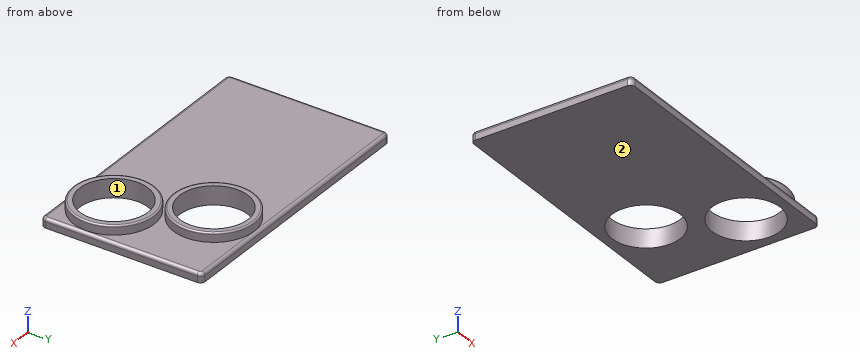
from build123d import *

# Parameters (mm, degrees)
F0_R         = 82.55
F0_R_2       = 69.85
F1_DEPTH     = 38.1
F0_W         = 558.8
F0_H         = 330.2
F2_DEPTH     = 19.05
F3_R         = 6.34999
F4_T1_DEPTH  = 42.8625
F4_T4_ANGLE  = 90
F4_T6_ANGLE  = 90
F4_T8_ANGLE  = 90
F4_T10_ANGLE = 90
F5_R         = 3.175


# Not quite as in the source:
# - a fillet or chamfer that OpenCascade refuses, or shapes differently, is made with other operations: its cross-section is extruded or revolved along the edge and cut away or added
# - a fillet or chamfer is up to 0.001 mm smaller than in the source, because OpenCascade refuses the exact size


with BuildPart() as f1:
    # F0 (on Top) → F1 (new body)
    with BuildSketch(Plane.XY):
        with Locations((393.7, 241.3)):
            Circle(F0_R)
        with Locations((393.7, 241.3)):
            Circle(F0_R_2, mode=Mode.SUBTRACT)
    extrude(amount=F1_DEPTH)



with BuildPart() as f1b:
    # F0 (on Top) → F1, piece 2 (new body)
    with BuildSketch(Plane.XY):
        with Locations((469.9, 88.9)):
            Circle(F0_R)
        with Locations((469.9, 88.9)):
            Circle(F0_R_2, mode=Mode.SUBTRACT)
    extrude(amount=F1_DEPTH)


with BuildPart() as f1_1:
    add(f1.part)

    add(f1b.part)  # F2 merges F1b
    # F0 (on Top) → F2 (join)
    with BuildSketch(Plane.XY):
        with Locations((279.4, 165.1)):
            Rectangle(F0_W, F0_H)
        with Locations((469.9, 88.9)):
            Circle(F0_R, mode=Mode.SUBTRACT)
        with Locations((393.7, 241.3)):
            Circle(F0_R, mode=Mode.SUBTRACT)
    extrude(amount=F2_DEPTH)

    # F3 (radius 6.35 in the source; OpenCascade refuses exactly that, so slightly less here)
    f3_edges = [f1_1.edges().sort_by_distance(p)[0] for p in [
        (0, 165.1, 19.05),
        (279.4, 330.2, 19.05),
        (279.4, 0, 19.05),
        (558.8, 165.1, 19.05),
    ]]
    fillet(f3_edges, radius=F3_R)

    # F4: fillet of radius 9.525 on 4 edges, made by hand

    # F4_s2 → F4_t1 (cut)
    with BuildSketch(Plane.XY.offset(-23.8125)):
        with BuildLine():
            ThreePointArc((0, 9.525), (2.7898079092, 2.7898079092), (9.525, 0))
            Line((9.525, 0), (0, 0))
            Line((0, 0), (0, 9.525))
        make_face()
        with BuildLine():
            ThreePointArc((549.275, 0), (556.0101920908, 2.7898079092), (558.8, 9.525))
            Line((558.8, 9.525), (558.8, 0))
            Line((558.8, 0), (549.275, 0))
        make_face()
        with BuildLine():
            ThreePointArc((549.275, 330.2), (556.0101920908, 327.4101920908), (558.8, 320.675))
            Line((558.8, 320.675), (558.8, 330.2))
            Line((558.8, 330.2), (549.275, 330.2))
        make_face()
        with BuildLine():
            ThreePointArc((0, 320.675), (2.7898079092, 327.4101920908), (9.525, 330.2))
            Line((9.525, 330.2), (0, 330.2))
            Line((0, 330.2), (0, 320.675))
        make_face()
    extrude(amount=F4_T1_DEPTH, mode=Mode.SUBTRACT)

    # F4_s3 → F4_t4 (revolve, cut)
    with BuildSketch(Plane.YZ.offset(9.525)):
        with BuildLine():
            ThreePointArc((323.85001, 19.05), (328.3401309895, 17.1901309895), (330.2, 12.70001))
            Line((330.2, 12.70001), (330.2, 19.05))
            Line((330.2, 19.05), (323.85001, 19.05))
        make_face()
    revolve(axis=Axis((9.525, 320.675, 19.05), (0, 0, 1)), revolution_arc=F4_T4_ANGLE, mode=Mode.SUBTRACT)

    # F4_s5 → F4_t6 (revolve, cut)
    with BuildSketch(Plane.XZ.offset(-320.675)):
        with BuildLine():
            ThreePointArc((552.45001, 19.05), (556.9401309895, 17.1901309895), (558.8, 12.70001))
            Line((558.8, 12.70001), (558.8, 19.05))
            Line((558.8, 19.05), (552.45001, 19.05))
        make_face()
    revolve(axis=Axis((549.275, 320.675, 19.05), (0, 0, 1)), revolution_arc=F4_T6_ANGLE, mode=Mode.SUBTRACT)

    # F4_s7 → F4_t8 (revolve, cut)
    with BuildSketch(Plane.YZ.offset(549.275)):
        with BuildLine():
            ThreePointArc((6.34999, 19.05), (1.8598690105, 17.1901309895), (0, 12.70001))
            Line((0, 12.70001), (0, 19.05))
            Line((0, 19.05), (6.34999, 19.05))
        make_face()
    revolve(axis=Axis((549.275, 9.525, 19.05), (0, 0, 1)), revolution_arc=F4_T8_ANGLE, mode=Mode.SUBTRACT)

    # F4_s9 → F4_t10 (revolve, cut)
    with BuildSketch(Plane.XZ.offset(-9.525)):
        with BuildLine():
            ThreePointArc((6.34999, 19.05), (1.8598690105, 17.1901309895), (0, 12.70001))
            Line((0, 12.70001), (0, 19.05))
            Line((0, 19.05), (6.34999, 19.05))
        make_face()
    revolve(axis=Axis((9.525, 9.525, 19.05), (0, 0, 1)), revolution_arc=F4_T10_ANGLE, mode=Mode.SUBTRACT)

    # F5
    f5_edges = [f1_1.edges().sort_by_distance(p)[0] for p in [
        (387.35, 88.9, 38.1),
        (311.15, 241.3, 38.1),
    ]]
    fillet(f5_edges, radius=F5_R)


solid = f1_1.part
Work out the finished part from the listing and answer in its coordinate system (mm). Face numbers are marked on the shaded views. Coordinates: 2 decimals unless noted, no trailing zeros. Write each loop counter-clockwise with the first axis right and the second up, starting at its lowest first coordinate (ties: lowest second). Pieces come first, ordered by that corner, then holes.
1. Consider line 1 along X through (y, z) = (238.5, 20); line 2 along Y through (x, z) = (393.7, 24); line 3 along Z through (x, y) = (337, 123.5). Determine where each line is inside the solid, lowest interval first.
Results list:
line 1: x = 311.2 to 323.91, 463.49 to 476.2
line 2: y = 57.15 to 120.65, 158.75 to 171.45, 311.15 to 323.85
line 3: z = 0 to 19.05
2. The part is cut by section C-C, the plane x = 38.5. Write down the section's boundary in (y, z), and give its area (3 significant figures).
Results list:
outline: (0, 0) - (330.2, 0) - (330.2, 12.7) arc R6.35 ccw to (323.85, 19.05) - (6.35, 19.05) arc R6.35 ccw to (0, 12.7) - close
area: 6,270 mm2
3. For a pull along X with two mould halves and no side action, classify the marked faces 1 and 2 as +X half, -X half, draft (parallel to the pull), parting line (faces both ways), or undercut.
Results list:
face 1: undercut
face 2: draft
4. Flat-ended cylindrical pins translate along their axes: pin 1 (1 mm diameter, centred on x = 176, z = 14, fed in from +Y); pin 2 (2 mm diameter, centred on y = 230.5, z = 28, fed in from -X); pin 3 (3 mm diameter, centred on x = 350.5, z = 17.5, fed in from -Y); pin 4 (5 mm diameter, centred on x = 190.5, z = 24, fed in from +Y). Find the tip coordinate at first contact, or state that the pin passes through.
Results list:
pin 1: stops at y = 330.15
pin 2: stops at x = 311.73
pin 3: stops at y = 0.92
pin 4: passes through
5. The part is cut by section A-A, the plane y = 241.3. Write down the section's boundary in (x, z) (3 decimals), and give its area (3 significant figures).
Results list:
outline: (0, 0) - (323.85, 0) - (323.85, 38.1) - (314.325, 38.1) arc R3.175 ccw to (311.15, 34.925) - (311.15, 19.05) - (6.35, 19.05) arc R6.35 ccw to (0, 12.7) - close; (463.55, 0) - (558.8, 0) - (558.8, 12.7) arc R6.35 ccw to (552.45, 19.05) - (476.25, 19.05) - (476.25, 34.925) arc R3.175 ccw to (473.075, 38.1) - (463.55, 38.1) - close
area: 8,450 mm2
6. The part is cut by section B-B, the plane z = 6. Write down the section's boundary in (x, y) (3 decimals).
Results list:
outline: (0, 9.525) arc R9.525 ccw to (9.525, 0) - (549.275, 0) arc R9.525 ccw to (558.8, 9.525) - (558.8, 320.675) arc R9.525 ccw to (549.275, 330.2) - (9.525, 330.2) arc R9.525 ccw to (0, 320.675) - close; hole circle Ø139.7 at (393.7, 241.3); hole circle Ø139.7 at (469.9, 88.9)
7. The part is cut by section D-D, the plane x = 448. State how many separate pieces and enclosed holes the cut face has, and give its area (3 significant figures).
Results list:
separate pieces: 3
enclosed holes: 0
area: 3,260 mm2
